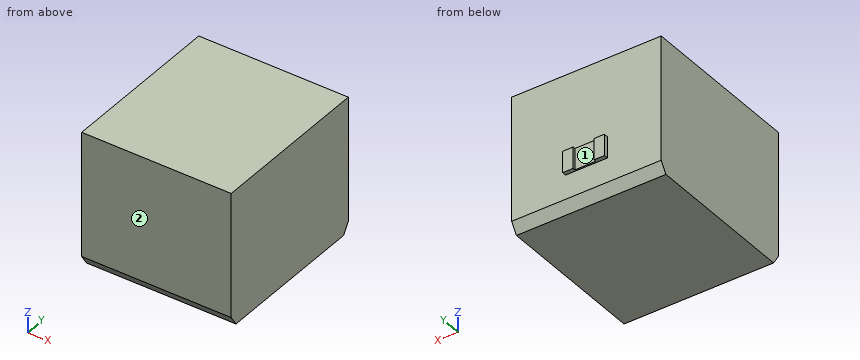
```python
from build123d import *

# Parameters (mm, degrees)
BOSS_EXTRUDE1_DEPTH  = 1016
SKETCH2_W            = 834.909944441
SKETCH2_H            = 965.348785231
CUT_EXTRUDE1_DEPTH   = 723.9
SKETCH3_R            = 38.1
BOSS_EXTRUDE2_DEPTH  = 723.9
SKETCH4_R            = 21.824467542
BOSS_EXTRUDE3_DEPTH  = 3.556
LPATTERN4_COUNT      = 7
LPATTERN4_PITCH      = 114.3
LPATTERN4_COUNT_DIR2 = 9
LPATTERN4_PITCH_DIR2 = 104.14
BOSS_EXTRUDE5_REACH  = 1421.937
SKETCH5_W            = 25.790965235
SKETCH5_H            = 508
SKETCH6_W            = 255.319328018
SKETCH6_H            = 131.057449743
BOSS_EXTRUDE6_DEPTH  = 10.16
SKETCH7_W            = 63.5
SKETCH7_H            = 131.057449743
BOSS_EXTRUDE7_DEPTH  = 15.24


with BuildPart() as part:
    # Sketch1 → Boss-Extrude1 (new body)
    with BuildSketch(Plane(origin=(0, 0, 0), x_dir=(1, 0, 0), z_dir=(0, 1, 0))):
        Polygon((-457.2, -381), (-457.2, 381), (457.2, 380.492), (457.2, -380.492), align=None)
    extrude(amount=BOSS_EXTRUDE1_DEPTH)

    # Sketch2 → Cut-Extrude1 (cut)
    with BuildSketch(Plane(origin=(0.21152549, 0, -380.745882486), x_dir=(-0.9999998456790481, 0, -0.0005555554698215814), z_dir=(0.0005555554698215814, 0, -0.9999998456790481))):
        with Locations((0.106508893, 511.58382344)):
            Rectangle(SKETCH2_W, SKETCH2_H)
    extrude(amount=-CUT_EXTRUDE1_DEPTH, mode=Mode.SUBTRACT)

    # Sketch3 → Boss-Extrude2 (add)
    with BuildSketch(Plane(origin=(-0.190641114, 0, 343.154005801), x_dir=(-0.9999998456790481, 0, -0.0005555554698216001), z_dir=(0.0005555554698216001, 0, -0.9999998456790481))):
        with Locations((-351.253434757, 946.469423659)):
            Circle(SKETCH3_R)
    boss_extrude2 = extrude(amount=BOSS_EXTRUDE2_DEPTH)

    # Sketch4 → Boss-Extrude3 (add)
    with BuildSketch(Plane(origin=(0.21152549, 0, -380.745882486), x_dir=(-0.9999998456790481, 0, -0.0005555554698216001), z_dir=(0.0005555554698216001, 0, -0.9999998456790481))):
        with Locations((-354.287460121, 946.233273052)):
            Circle(SKETCH4_R)
    boss_extrude3 = extrude(amount=BOSS_EXTRUDE3_DEPTH)

    # LPattern4: Boss-Extrude2, Boss-Extrude3 7 × 9
    with Locations(*[Vector(-0.9999998456790481, 0, -0.0005555554698216149) * (i * LPATTERN4_PITCH) + Vector(0, -1, 0) * (j * LPATTERN4_PITCH_DIR2) for i in range(LPATTERN4_COUNT) for j in range(LPATTERN4_COUNT_DIR2) if (i, j) != (0, 0)]):
        add(boss_extrude2)
        add(boss_extrude3)

    # Boss-Extrude5: up to this face of the body (flat: up to its plane)
    boss_extrude5_end = Plane(part.part.faces().sort_by_distance((457.2, 508, 0))[0])
    # Sketch5 → Boss-Extrude5 (add, up to the picked face)
    with BuildSketch(Plane.ZY.offset(457.2), mode=Mode.PRIVATE) as boss_extrude5_sk1:
        with Locations((-368.104517383, 254)):
            Rectangle(SKETCH5_W, SKETCH5_H)
    boss_extrude5_tool1 = split(extrude(boss_extrude5_sk1.sketch, amount=-BOSS_EXTRUDE5_REACH, mode=Mode.PRIVATE), bisect_by=boss_extrude5_end, keep=Keep.BOTH, mode=Mode.PRIVATE)
    # Sketch5 → Boss-Extrude5 (add, up to the picked face)
    with BuildSketch(Plane.ZY.offset(457.2), mode=Mode.PRIVATE) as boss_extrude5_sk2:
        with Locations((-368.104517383, 762)):
            Rectangle(SKETCH5_W, SKETCH5_H)
    boss_extrude5_tool2 = split(extrude(boss_extrude5_sk2.sketch, amount=-BOSS_EXTRUDE5_REACH, mode=Mode.PRIVATE), bisect_by=boss_extrude5_end, keep=Keep.BOTH, mode=Mode.PRIVATE)
    # Sketch5 → Boss-Extrude5 (add, up to the picked face)
    with BuildSketch(Plane.ZY.offset(457.2), mode=Mode.PRIVATE) as boss_extrude5_sk3:
        Polygon((-444.109034765, 41.018337697), (-381, 0), (-381, 508), (-444.109034765, 508), align=None)
    boss_extrude5_tool3 = split(extrude(boss_extrude5_sk3.sketch, amount=-BOSS_EXTRUDE5_REACH, mode=Mode.PRIVATE), bisect_by=boss_extrude5_end, keep=Keep.BOTH, mode=Mode.PRIVATE)
    # Sketch5 → Boss-Extrude5 (add, up to the picked face)
    with BuildSketch(Plane.ZY.offset(457.2), mode=Mode.PRIVATE) as boss_extrude5_sk4:
        Polygon((-444.109034765, 508), (-381, 508), (-381, 1016), (-444.109034765, 974.981662303), align=None)
    boss_extrude5_tool4 = split(extrude(boss_extrude5_sk4.sketch, amount=-BOSS_EXTRUDE5_REACH, mode=Mode.PRIVATE), bisect_by=boss_extrude5_end, keep=Keep.BOTH, mode=Mode.PRIVATE)
    add(boss_extrude5_tool1.solids().sort_by(Axis((-457.2, 254, -368.104517), (1, 0, 0)))[0])
    add(boss_extrude5_tool2.solids().sort_by(Axis((-457.2, 762, -368.104517), (1, 0, 0)))[0])
    add(boss_extrude5_tool3.solids().sort_by(Axis((-457.2, 264.110778, -412.112009), (1, 0, 0)))[0])
    add(boss_extrude5_tool4.solids().sort_by(Axis((-457.2, 751.889222, -412.112009), (1, 0, 0)))[0])

    # Sketch6 → Boss-Extrude6 (add)
    with BuildSketch(Plane(origin=(0, 1016, 0), x_dir=(1, 0, 0), z_dir=(0, 1, 0))):
        with Locations((0, 166.980548784)):
            Rectangle(SKETCH6_W, SKETCH6_H)
    extrude(amount=BOSS_EXTRUDE6_DEPTH)

    # Sketch7 → Boss-Extrude7 (add)
    with BuildSketch(Plane(origin=(0, 1026.16, 0), x_dir=(1, 0, 0), z_dir=(0, 1, 0))):
        with Locations((-95.909664009, 166.980548784)):
            Rectangle(SKETCH7_W, SKETCH7_H)
        with Locations((95.909664009, 166.980548784)):
            Rectangle(SKETCH7_W, SKETCH7_H)
    extrude(amount=BOSS_EXTRUDE7_DEPTH)


solid = part.part
```
Verification items for the finished model (mm, model axes). Face numbers are marked on the shaded views. A direction names the side the tool comes from. Coordinates: 2 decimals unless noted, no trailing zeros. Loops run counter-clockwise (first coordinate to the right, second up) from the corner with the lowest first, then second, coordinate; pieces in that order, holes last. Notation, with made-up numbers: (1, -18.75) - (27, -18.75) arc R32 cw to (27, 18.25) - close; hole circle Ø7 at (45.25, 11.25). An arc over 180 degrees is marked (long way). Return JSON: item names as keys, results as strings.
1. Go/stop test with flat-tipped pins: pin 1 (7.5 mm diameter, centred on y = 1030.5, z = -163.5, fed in from +X); pin 2 (12 mm diameter, centred on y = 1037.5, z = -150.5, fed in from -X); pin 3 (12.5 mm diameter, centred on x = 38, y = 1024.5, fed in from -Z). Record where each tip stops, or that it passes through.
Established:
{"pin 1": "stops at x = 127.66", "pin 2": "stops at x = -127.66", "pin 3": "stops at z = -232.51"}
2. Thickness scan on L1, parallel to Z at x = -66, y = 795; L2, parallel to Z at x = -402, y = 128; L3, parallel to Y at x = 163.5, z = -272.5. Record the ranges inside material, lowest first.
Established:
{"L1": "z = -444.11 to -355.21, 343.12 to 380.78", "L2": "z = -444.11 to -355.21, 342.93 to 380.97", "L3": "y = 0 to 28.91, 994.26 to 1016"}
3. Tool access check on the marked faces 1 and 2. Record the directions out of +Z, -Z, +X, -X, +Y, -Y that give a thin tool (end or side, any length) a straight path to the whole face; none if there is none.
Established:
{"face 1": "+Z, -Z, +Y", "face 2": "+Z, -Z, +X, -X, -Y"}
4. Section check B-B, the plane x = 289. Record the boundary of the cut face in (y, z), then the cut area to 3 significant figures.
Established:
{"outline": "(0, -381) - (41.02, -444.11) - (974.98, -444.11) - (1016, -381) - (1016, 380.59) - (0, 380.59) - close; hole (28.91, -355.21) - (994.26, -355.21) - (994.26, 343.31) - (28.91, 343.31) - close", "area": "161,000 mm2"}
5. Section check A-A, the plane z = 176. Count the separate pieces of the cut face and the enclosed holes in it, then the cut area to 3 significant figures.
Established:
{"separate pieces": "64", "enclosed holes": "1", "area": "410,000 mm2"}
